Model file for the job. Use its own axes, mm. A direction names the side the tool comes from. Round coordinates to 2 decimals unless told otherwise and drop trailing zeros. Order: outer loops, then holes, each group sorted by start corner. A loop starts at its lowest first (then second) coordinate and runs counter-clockwise, first axis right, second up. Notation, with made-up numbers: (-30, -3) - (-6, -3) arc R4 ccw to (-6, 1) - close; hole circle Ø8 at (54, -0.75). An arc over 180 degrees is marked (long way). Answer as CSV lines item,"result". Start each with the question number.
1. Band-saw the part on C-C on z = 1.95. List the corners of the cut face in (x, y).
2. Wall check: line 1 along Y through (x, z) = (30, 0.2); line 2 along Y through (x, z) = (30, 2.9); line 3 along X through (y, z) = (8.75, 3.3). Give the ranges that are in metal, low to high. Write a range as [from, to].
3. Band-saw the part on A-A on x = -3. List the corners of the cut face in (y, z), then the cut area to 3 significant figures.
4. 3-axis set-ups, long thin cutter, end or side, ignore diameter. For faces 5 (the face through (32.5, -6.1, 2.2)), 6 (the face through (-10, 3, 5)), 7 (the face through (30, 0, 0.5)), 8 (the face through (-11, 0, 3)), 9 (the face through (6.9, 4.5, 5.5)): which of +Z, -Z, +X, -X, +Y, -Y reach the whole face in a straight line?
5. Band-saw the part on D-D on x = 30. List the corners of the cut face in (y, z), then the cut area to 3 significant figures.
6. Band-saw the part on B-B on y = 6. List the corners of the cut face in (x, z).
7. Pull direction Y, two halves, no side cores. Call faces 1 (the face through (14, 3, 5.5)), 2 (the face through (-9.5, 8.5, 5.5)), 3 (the face through (15, -12.5, 3)), 4 (the face through (32, 0, 4)): released by +Y, released by -Y, zero draft, split by the parting line, or undercut.
8. Pin check, flat tips, straight feed: pin 1 Ø2.5 at (x, y) = (-9.5, 2.5) entering from +Z; pin 2 Ø1 at (x, y) = (7.5, -6) entering from -Z; pin 3 Ø7 at (x, y) = (30, 6) entering from +Z. Stop position of each tip, or through.
```python
from build123d import *

# Parameters (mm, degrees)
SKETCH1_W           = 40
SKETCH1_H           = 25
BOSS_EXTRUDE1_DEPTH = 6
CUT_EXTRUDE1_START  = 6
SKETCH3_W           = 14
SKETCH3_H           = 3
SKETCH3_W_2         = 3
SKETCH3_H_2         = 11
CUT_EXTRUDE1_DEPTH  = 1
SKETCH4_R           = 1.4
CUT_EXTRUDE2_DEPTH  = 11
SKETCH7_W           = 9
SKETCH7_H           = 25
CUT_EXTRUDE5_DEPTH  = 21
SKETCH8_W           = 20
SKETCH8_H           = 25
BOSS_EXTRUDE2_DEPTH = 4
SKETCH9_R           = 2.5
CUT_EXTRUDE6_DEPTH  = 43.334973721
CUT_EXTRUDE7_DEPTH  = 0.5
FILLET3_R           = 1
FILLET4_R           = 5
FILLET5_R           = 5


with BuildPart() as part:
    # Sketch1 → Boss-Extrude1 (new body)
    with BuildSketch(Plane.XY):
        Rectangle(SKETCH1_W, SKETCH1_H)
    extrude(amount=BOSS_EXTRUDE1_DEPTH)

    # Sketch3 → Cut-Extrude1 (cut)
    with BuildSketch(Plane.XY.offset(CUT_EXTRUDE1_START)):
        with Locations((7, 3)):
            Rectangle(SKETCH3_W, SKETCH3_H)
        with Locations((-9.5, 3)):
            Rectangle(SKETCH3_W_2, SKETCH3_H_2)
    extrude(amount=-CUT_EXTRUDE1_DEPTH, mode=Mode.SUBTRACT)

    # Sketch4 → Cut-Extrude2 (cut)
    with BuildSketch(Plane.XY):
        with Locations(Location((16, 9, 0), (0, 0, 180))):
            Circle(SKETCH4_R)
        with Locations(Location((-3, 9, 0), (0, 0, 180))):
            Circle(SKETCH4_R)
    extrude(amount=CUT_EXTRUDE2_DEPTH, mode=Mode.SUBTRACT)

    # Sketch7 → Cut-Extrude5 (cut)
    with BuildSketch(Plane.XY):
        with Locations((-15.5, 0)):
            Rectangle(SKETCH7_W, SKETCH7_H)
    extrude(amount=CUT_EXTRUDE5_DEPTH, mode=Mode.SUBTRACT)

    # Sketch8 → Boss-Extrude2 (add)
    with BuildSketch(Plane.XY):
        with Locations((30, 0)):
            Rectangle(SKETCH8_W, SKETCH8_H)
    extrude(amount=BOSS_EXTRUDE2_DEPTH)

    # Sketch9 → Cut-Extrude6 (cut, through all)
    with BuildSketch(Plane.XY):
        with Locations((30, 6)):
            Circle(SKETCH9_R)
        with Locations(Location((30, -6, 0), (0, 0, 180))):
            Circle(SKETCH9_R)
    extrude(amount=CUT_EXTRUDE6_DEPTH, mode=Mode.SUBTRACT)

    # Sketch10 → Cut-Extrude7 (cut)
    with BuildSketch(Plane.XY):
        with BuildLine():
            Line((27.452141011, -0.567835185), (27.452141011, 0.567835185))
            ThreePointArc((27.452141011, 0.567835185), (29.956756767, 11.999844167), (32.625893719, 0.605124452))
            Line((32.625893719, 0.605124452), (32.625893719, 0.058283872))
            Line((32.625893719, 0.058283872), (32.625893719, -0.605124452))
            ThreePointArc((32.625893719, -0.605124452), (29.956756767, -11.999844167), (27.452141011, -0.567835185))
        make_face()
    extrude(amount=CUT_EXTRUDE7_DEPTH, mode=Mode.SUBTRACT)

    # Fillet3
    # the kernel refuses this fillet: 1 mm, written as the material it takes off along each edge
    with BuildSketch(Plane(origin=(27.452141011, -0.567835185, -1.505321413), x_dir=(-0.8846564558137137, -0.466243450556808, 0), z_dir=(0, 0, 1))) as fillet3_piece_1:
        with BuildLine():
            CenterArc((0.603917956, -0.998920373), FILLET3_R, 92.662646755, 59.546627489)
            Line((-0.2807385, -0.532676923), (0, 0))
            ThreePointArc((0, 0), (0.278731364, -0.006477761), (0.557462728, 0))
        make_face()
    extrude(amount=2.005321413, mode=Mode.SUBTRACT)
    with BuildSketch(Plane(origin=(27.452141011, 0.567835185, -1.505321413), x_dir=(-0.8846564558137143, 0.46624345055680716, 0), z_dir=(0, 0, 1))) as fillet3_piece_2:
        with BuildLine():
            CenterArc((0.603917956, 0.998920373), FILLET3_R, 207.790725756, 59.546627489)
            Line((-0.2807385, 0.532676923), (0, 0))
            ThreePointArc((0, 0), (0.278731364, 0.006477761), (0.557462728, 0))
        make_face()
    extrude(amount=2.005321413, mode=Mode.SUBTRACT)
    with BuildSketch(Plane(origin=(32.625893719, -0.605124452, -1.482132829), x_dir=(0.8781869817379448, -0.4783174940413514, 0), z_dir=(0, 0, 1))) as fillet3_piece_3:
        with BuildLine():
            CenterArc((0.594614958, 0.998953396), FILLET3_R, 208.575572443, 58.80282617)
            Line((-0.283572024, 0.520635902), (0, 0))
            ThreePointArc((0, 0), (0.274437673, 0.006279622), (0.548875345, 0))
        make_face()
    extrude(amount=1.982132829, mode=Mode.SUBTRACT)
    with BuildSketch(Plane(origin=(32.625893719, 0.605124452, -1.482132829), x_dir=(0, -1, 0), z_dir=(0, 0, 1))) as fillet3_piece_4:
        with BuildLine():
            CenterArc((0.592853132, 1), FILLET3_R, 211.19717383, 58.80282617)
            ThreePointArc((-0.26253668, 0.482015183), (-0.125753657, 0.244011245), (0, 0))
            Line((0, 0), (0.592853132, 0))
        make_face()
    extrude(amount=1.982132829, mode=Mode.SUBTRACT)

    # Fillet4
    # the kernel refuses this fillet: 5 mm, written as the material it adds along each edge
    with BuildSketch(Plane(origin=(20, -12.5, 4), x_dir=(0, 0, 1), z_dir=(0, 1, 0))) as fillet4_piece_1:
        with BuildLine():
            CenterArc((5, 4), FILLET4_R, 180, 53.130102354)
            Line((0, 4), (-0.1, 4))
            Line((-0.1, 4), (-0.1, 0))
            Line((-0.1, 0), (0, -0.1))
            ThreePointArc((0, -0.1), (1, -0.1), (1.94, -0.08))
            Line((1.94, -0.08), (2, 0))
        make_face()
    extrude(amount=25)

    # Fillet5
    fillet5_edges = [part.edges().sort_by_distance(p)[0] for p in [
        (20, 0, 6),
    ]]
    fillet(fillet5_edges, radius=FILLET5_R)


solid = part.part
```
Reply:
1,outline,"(-11, -12.5) - (40, -12.5) - (40, 12.5) - (-11, 12.5) - close; hole circle Ø2.8 at (-3, 9); hole circle Ø2.8 at (16, 9); hole circle Ø5 at (30, -6); hole circle Ø5 at (30, 6)"
2,line 1,"y = [-12.5, -12], [12, 12.5]"
2,line 2,"y = [-12.5, -8.5], [-3.5, 3.5], [8.5, 12.5]"
2,line 3,"x = [-11, -4.38], [-1.62, 14.62], [17.38, 40]"
3,outline,"(-12.5, 0) - (7.6, 0) - (7.6, 6) - (-12.5, 6) - close; (10.4, 0) - (12.5, 0) - (12.5, 6) - (10.4, 6) - close"
3,area,"133 mm2"
4,face 5,"+Z, -Z"
4,face 6,"+Z, -X"
4,face 7,"-Z"
4,face 8,"+Z, -Z, -X, +Y, -Y"
4,face 9,"+Z"
5,outline,"(-12.5, 0) - (-12, 0) - (-12, 0.5) - (-8.5, 0.5) - (-8.5, 4) - (-12.5, 4) - close; (-3.5, 0.5) - (3.5, 0.5) - (3.5, 4) - (-3.5, 4) - close; (8.5, 0.5) - (12, 0.5) - (12, 0) - (12.5, 0) - (12.5, 4) - (8.5, 4) - close"
5,area,"53.0 mm2"
6,outline,"(-11, 0) - (24, 0) - (24, 0.5) - (27.5, 0.5) - (27.5, 4) - (24, 4) arc R5 cw to (21, 5) arc R5 ccw to (18, 6) - (-8, 6) - (-8, 5) - (-11, 5) - close; (32.5, 0.5) - (36, 0.5) - (36, 0) - (40, 0) - (40, 4) - (32.5, 4) - close"
7,face 1,"undercut"
7,face 2,"undercut"
7,face 3,"released by -Y"
7,face 4,"zero draft"
8,pin 1,"stops at z = 5"
8,pin 2,"stops at z = 0"
8,pin 3,"stops at z = 4"
